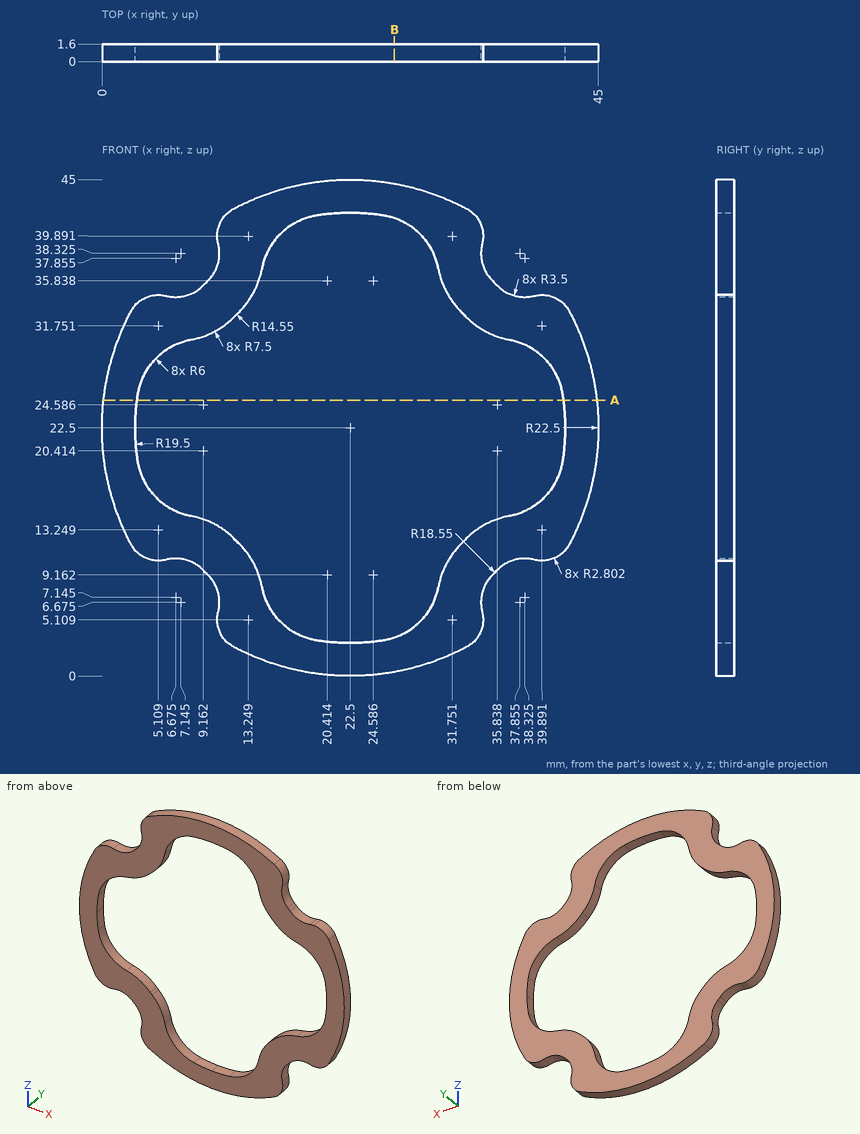
Part print with two shaded views. Sizes in mm from the minimum x, y, z corner. Coordinates: 2 decimals unless noted, no trailing zeros. Order: outer loops, then holes, each group sorted by start corner. A loop starts at its lowest first (then second) coordinate and runs counter-clockwise, first axis right, second up. Notation, with made-up numbers: (21, 49.25) - (69, 49.25) arc R23 cw to (69, 75.25) - close; hole circle Ø11 at (81.5, -4.75). An arc over 180 degrees is marked (long way). Write item = value, one per line. Start each with the question number.
1) Saw through at A-A on z = 25. Write the cut outline in (x, y).
2) Wall check: line 1 along X through (y, z) = (1.25, 22) (1 decimal); line 2 along Z through (x, y) = (17.5, 1.2); line 3 along Z through (x, y) = (8, 0.3) (1 decimal). Give the ranges that are in metal, low to high. Write a range as from..to.
3) Saw through at B-B on x = 26.5. Write the cut outline in (y, z) (1 decimal).
4) Flat gauge pins, fed straight in: pin 1 Ø8 at (x, z) = (32, 9.5) entering from -Y; pin 2 Ø8 at (x, z) = (17.5, 29.5) entering from +Y. Where does each tip first touch, or does it go through?
From the geometry:
q1.outline = (0.14, 0) - (3.16, 0) - (3.16, 1.6) - (0.14, 1.6) - close; (41.84, 0) - (44.86, 0) - (44.86, 1.6) - (41.84, 1.6) - close
q2.line_1 = 0..3, 42..45
q2.line_2 = 0.56..3.92, 41.08..44.44
q2.line_3 = 10.4..14.5, 30.5..34.6
q3.outline = (0, 0.4) - (1.6, 0.4) - (1.6, 3.5) - (0, 3.5) - close; (0, 41.5) - (1.6, 41.5) - (1.6, 44.6) - (0, 44.6) - close
q4.pin_1 = 0
q4.pin_2 = through
